Here's how the part is built. I have some questions about the finished solid (model axes, mm). Round coordinates to 2 decimals unless told otherwise and drop trailing zeros. Loops run counter-clockwise (first coordinate to the right, second up) from the corner with the lowest first, then second, coordinate; pieces in that order, holes last. Notation, with made-up numbers: (-12, 63) - (21, 63) arc R7 cw to (21, 71) - close; hole circle Ø7 at (50.5, -17.5). An arc over 180 degrees is marked (long way). Answer as a JSON object with one key per item and string values. Group by question number.
1) I want a section at B-B, the plane x = 2. Please give me the cut outline in (y, z).
2) I want a section at A-A, the plane y = -3. Please give me the cut outline in (x, z), then the cut area to 3 significant figures.
3) I want a section at D-D, the plane y = 21.5. Please give me the cut outline in (x, z).
4) I want a section at C-C, the plane z = 23.5. Please give me the cut outline in (x, y).
5) If I drill on line 1 along Y through (x, z) = (0.7, -55); line 2 along Z through (x, y) = (0.4, -1); line 3 along Y through (x, z) = (2.4, 38.5), over which ranges is the centre line in solid material (lowest first)? Write a range as [from, to].
Autodesk Inventor part; units mm, degrees
ref_plane "YZ Plane" through (0, 0, 0) normal (1, 0, 0) x (0, 1, 0)
ref_plane "XZ Plane" through (0, 0, 0) normal (0, 1, 0) x (-1, 0, 0)
ref_plane "XY Plane" through (0, 0, 0) normal (0, 0, 1) x (1, 0, 0)
sketch "Sketch1" plane through (0, 0, 0) normal (1, 0, 0) x (0, 1, 0)
  line L0 (0, 55.6574) -> (32.5774, -33.8483)
  line L1 (0, 55.6574) -> (-7.62, 55.6574)
  line L2 (-7.62, 55.6574) -> (-7.62, -33.8483)
  line L3 (32.5774, -33.8483) -> (32.5774, -71.9483)
  line L4 (32.5774, -71.9483) -> (-7.62, -71.9483)
  line L5 (-7.62, -71.9483) -> (-7.62, -33.8483)
  point P0 (0, 0)
  dimension "d1" = 95.25
  dimension "d4" = 20
  dimension "d5" = 7.62
  dimension "d6" = 38.1
extrude "Extrusion1" add sketch "Sketch1" along normal blind 2.54
sketch "Sketch2" plane through (2.54, 0, 0) normal (1, 0, 0) x (0, 0, -1)
  line L0 (48.7581, 6.223) -> (60.9501, 6.223)
  line L1 (60.9501, 6.223) -> (60.9501, -4.8514)
  line L2 (60.9501, -4.8514) -> (48.7581, -4.8514)
  line L3 (48.7581, -4.8514) -> (48.7581, 6.223)
  line L4 (-55.6574, -7.62) -> (71.9483, -7.62)
  line L5 (71.9483, -7.62) -> (71.9483, 32.5774)
  point P0 (0, 0)
  dimension "d7" = 12.192
  dimension "d8" = 11.0744
  dimension "d11" = 2.7686
  dimension "d12" = 10.9982
extrude "Extrusion2" cut sketch "Sketch2" against normal blind 2.54
properties part number "sideWithHole"
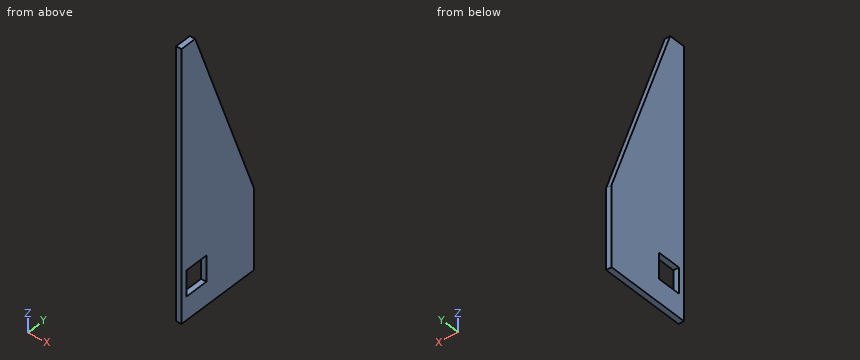
Outcome:
{
 "1": {"outline": "(-7.62, -71.95) - (32.58, -71.95) - (32.58, -33.85) - (0, 55.66) - (-7.62, 55.66) - close; hole (-4.85, -60.95) - (6.22, -60.95) - (6.22, -48.76) - (-4.85, -48.76) - close"},
 "2": {"outline": "(0, -71.95) - (2.54, -71.95) - (2.54, -60.95) - (0, -60.95) - close; (0, -48.76) - (2.54, -48.76) - (2.54, 55.66) - (0, 55.66) - close", "area": "293 mm^2"},
 "3": {"outline": "(0, -71.95) - (2.54, -71.95) - (2.54, -3.41) - (0, -3.41) - close"},
 "4": {"outline": "(0, -7.62) - (2.54, -7.62) - (2.54, 11.7) - (0, 11.7) - close"},
 "5": {"line 1": "[-7.62, -4.85], [6.22, 32.58]", "line 2": "[-71.95, -60.95], [-48.76, 55.66]", "line 3": "[-7.62, 6.24]"}
}
